Source: CAD feature listing. Evaluate the final solid. Frame: model axes, mm. A direction names the side the tool comes from. Give positions to 0.01 mm unless a question says otherwise; leave off trailing zeros. Order: outer loops, then holes, each group sorted by start corner. A loop starts at its lowest first (then second) coordinate and runs counter-clockwise, first axis right, second up.
from build123d import *

# Parameters (mm, degrees)
SKETCH1_W           = 50
SKETCH1_H           = 90
BOSS_EXTRUDE1_DEPTH = 10
SKETCH2_W           = 50
SKETCH2_H           = 50
SKETCH2_R           = 4.25
BOSS_EXTRUDE2_DEPTH = 10
SKETCH3_R           = 8.5
CUT_EXTRUDE1_DEPTH  = 5
CHAMFER1_SIZE       = 2


with BuildPart() as part:
    # Sketch1 → Boss-Extrude1 (new body)
    with BuildSketch(Plane(origin=(0, 0, 0), x_dir=(1, 0, 0), z_dir=(0, 1, 0))):
        with Locations((25, 45)):
            Rectangle(SKETCH1_W, SKETCH1_H)
        with BuildLine():
            Line((9, 6), (9, 84))
            ThreePointArc((9, 84), (12, 87), (15, 84))
            Line((15, 84), (15, 6))
            ThreePointArc((15, 6), (12, 3), (9, 6))
        make_face(mode=Mode.SUBTRACT)
        with BuildLine():
            Line((35, 6), (35, 84))
            ThreePointArc((35, 84), (38, 87), (41, 84))
            Line((41, 84), (41, 6))
            ThreePointArc((41, 6), (38, 3), (35, 6))
        make_face(mode=Mode.SUBTRACT)
    extrude(amount=BOSS_EXTRUDE1_DEPTH)

    # Sketch2 → Boss-Extrude2 (add)
    with BuildSketch(Plane.XY):
        with Locations((25, 25)):
            Rectangle(SKETCH2_W, SKETCH2_H)
        with Locations((25, 40)):
            Circle(SKETCH2_R, mode=Mode.SUBTRACT)
        with Locations((25, 20)):
            Circle(SKETCH2_R, mode=Mode.SUBTRACT)
    extrude(amount=BOSS_EXTRUDE2_DEPTH)

    # Sketch3 → Cut-Extrude1 (cut)
    with BuildSketch(Plane(origin=(0, 0, 0), x_dir=(-1, 0, 0), z_dir=(0, 0, -1))):
        with Locations((-25, 40)):
            Circle(SKETCH3_R)
        with Locations((-25, 20)):
            Circle(SKETCH3_R)
    extrude(amount=-CUT_EXTRUDE1_DEPTH, mode=Mode.SUBTRACT)

    # Chamfer1
    # the kernel refuses this chamfer: 2 mm, written as the material it takes off along each edge
    with BuildSketch(Plane(origin=(50, 10, 0), x_dir=(0.027495876610585623, -0.9996219169112968, 0), z_dir=(0, 0, -1))) as chamfer1_piece_1:
        Polygon((CHAMFER1_SIZE * 0.999621916911, CHAMFER1_SIZE * 0.0274958766106), (-CHAMFER1_SIZE * 0.0274958766106, CHAMFER1_SIZE * 0.999621916911), (0, 0), align=None)
    extrude(amount=95.143365976, mode=Mode.SUBTRACT)
    with BuildSketch(Plane(origin=(55.143365976, 10, -90), x_dir=(0, -0.9996219169112968, -0.027495876610589075), z_dir=(-1, 0, 0)), Plane(origin=(-5.143365976, 50, 0), x_dir=(0, 0.02749587661058563, 0.9996219169112968), z_dir=(1, 0, 0))) as chamfer1_piece_2:
        Polygon((CHAMFER1_SIZE * 0.999621916911, CHAMFER1_SIZE * 0.0274958766106), (-CHAMFER1_SIZE * 0.0274958766106, CHAMFER1_SIZE * 0.999621916911), (0, 0), align=None)
    extrude(amount=60.286731952, mode=Mode.SUBTRACT)
    with BuildSketch(Plane(origin=(50, 55.143365976, 0), x_dir=(0.02749587661058563, 0, 0.9996219169112968), z_dir=(0, -1, 0))) as chamfer1_piece_3:
        Polygon((CHAMFER1_SIZE * 0.999621916911, CHAMFER1_SIZE * 0.0274958766106), (-CHAMFER1_SIZE * 0.0274958766106, CHAMFER1_SIZE * 0.999621916911), (0, 0), align=None)
    extrude(amount=45.143365976, mode=Mode.SUBTRACT)
    with BuildSketch(Plane(origin=(0, 10, 0), x_dir=(0.9996219169112968, 0, -0.027495876610586372), z_dir=(0, 1, 0))) as chamfer1_piece_4:
        Polygon((CHAMFER1_SIZE * 0.999621916911, -CHAMFER1_SIZE * 0.0274958766106), (-CHAMFER1_SIZE * 0.0274958766106, -CHAMFER1_SIZE * 0.999621916911), (0, 0), align=None)
    extrude(amount=45.143365976, mode=Mode.SUBTRACT)
    with BuildSketch(Plane(origin=(0, 10, -95.143365976), x_dir=(0.9996219169112968, 0.027495876610586494, 0), z_dir=(0, 0, 1))) as chamfer1_piece_5:
        Polygon((CHAMFER1_SIZE * 0.999621916911, -CHAMFER1_SIZE * 0.0274958766106), (-CHAMFER1_SIZE * 0.0274958766106, -CHAMFER1_SIZE * 0.999621916911), (0, 0), align=None)
    extrude(amount=95.143365976, mode=Mode.SUBTRACT)
    with BuildSketch(Plane(origin=(50, 55.143365976, 0), x_dir=(0.02749587661058563, 0, 0.9996219169112968), z_dir=(0, -1, 0))) as chamfer1_piece_6a_section:
        Polygon((CHAMFER1_SIZE * 0.999621916911, CHAMFER1_SIZE * 0.0274958766106), (-CHAMFER1_SIZE * 0.0274958766106, CHAMFER1_SIZE * 0.999621916911), (0, 0), align=None)
    chamfer1_piece_6a = extrude(amount=50.286731952, mode=Mode.PRIVATE)
    chamfer1_piece_6a = split(chamfer1_piece_6a, bisect_by=Plane(origin=(49.340412746, 10, 0.659587254), z_dir=(0, -1, 0)), keep=Keep.TOP, mode=Mode.PRIVATE)
    with BuildSketch(Plane(origin=(50, 10, 5.143365976), x_dir=(0.027495876610585623, -0.9996219169112968, 0), z_dir=(0, 0, -1))) as chamfer1_piece_6b_section:
        Polygon((CHAMFER1_SIZE * 0.999621916911, CHAMFER1_SIZE * 0.0274958766106), (-CHAMFER1_SIZE * 0.0274958766106, CHAMFER1_SIZE * 0.999621916911), (0, 0), align=None)
    chamfer1_piece_6b = extrude(amount=100.286731952, mode=Mode.PRIVATE)
    chamfer1_piece_6b = split(chamfer1_piece_6b, bisect_by=Plane(origin=(49.340412746, 9.340412746, 0), z_dir=(0, 0, 1)), keep=Keep.TOP, mode=Mode.PRIVATE)
    chamfer1_piece_6 = chamfer1_piece_6a & chamfer1_piece_6b
    add(chamfer1_piece_6, mode=Mode.SUBTRACT)
    with BuildSketch(Plane(origin=(0, 4.856634024, 0), x_dir=(0.9996219169112968, 0, -0.027495876610586372), z_dir=(0, 1, 0))) as chamfer1_piece_7a_section:
        Polygon((CHAMFER1_SIZE * 0.999621916911, -CHAMFER1_SIZE * 0.0274958766106), (-CHAMFER1_SIZE * 0.0274958766106, -CHAMFER1_SIZE * 0.999621916911), (0, 0), align=None)
    chamfer1_piece_7a = extrude(amount=50.286731952, mode=Mode.PRIVATE)
    chamfer1_piece_7a = split(chamfer1_piece_7a, bisect_by=Plane(origin=(0.659587254, 10, 0.659587254), z_dir=(0, -1, 0)), keep=Keep.TOP, mode=Mode.PRIVATE)
    with BuildSketch(Plane(origin=(0, 10, -95.143365976), x_dir=(0.9996219169112968, 0.027495876610586494, 0), z_dir=(0, 0, 1))) as chamfer1_piece_7b_section:
        Polygon((CHAMFER1_SIZE * 0.999621916911, -CHAMFER1_SIZE * 0.0274958766106), (-CHAMFER1_SIZE * 0.0274958766106, -CHAMFER1_SIZE * 0.999621916911), (0, 0), align=None)
    chamfer1_piece_7b = extrude(amount=100.286731952, mode=Mode.PRIVATE)
    chamfer1_piece_7b = split(chamfer1_piece_7b, bisect_by=Plane(origin=(0.659587254, 9.340412746, 0), z_dir=(0, 0, 1)), keep=Keep.TOP, mode=Mode.PRIVATE)
    chamfer1_piece_7 = chamfer1_piece_7a & chamfer1_piece_7b
    add(chamfer1_piece_7, mode=Mode.SUBTRACT)


solid = part.part
1) First-contact query: pin 1 Ø10 at (x, y) = (25, 40) entering from +Z; pin 2 Ø14 at (x, z) = (27, -49.5) entering from +Y; pin 3 Ø8.5 at (x, y) = (22.5, 22.5) entering from -Z; pin 4 Ø5 at (y, z) = (11, -16.5) entering from -X. Flat tips, straight axial feed; report the tip coordinate or a pass-through.
Checks:
pin 1: stops at z = 10
pin 2: stops at y = 10
pin 3: stops at z = 5
pin 4: stops at x = 0.5
2) Reachability of faces 5 (the face through (38, 5, -3)), 6 (the face through (26.84, 11.7, 2.46)), 7 (the face through (25, 10, -45)) from +Z, -Z, +X, -X, +Y, -Y: full face, straight path, thin tool, end or side. Return the list, or none.
Checks:
face 5: +Y, -Y
face 6: -Z
face 7: -Z, +X, -X, +Y
3) Section query A-A on y = 5.5. Output: boundary loops of the cut face in (x, z), and give its area (3 significant figures).
Checks:
outline: (0, -90) - (50, -90) - (50, 10) - (0, 10) - close; hole (9, -84) arc R3 ccw to (15, -84) - (15, -6) arc R3 ccw to (9, -6) - close; hole (35, -84) arc R3 ccw to (41, -84) - (41, -6) arc R3 ccw to (35, -6) - close
area: 4,010 mm2
4) Ray query, L1, parallel to Y at x = 25, z = 6.4; L2, parallel to Y at x = 25, z = 2; L3, parallel to X at y = 40, z = 7. Return the intervals inside material, ascending.
Checks:
L1: y = 0 to 15.75, 24.25 to 35.75, 44.25 to 50
L2: y = 0 to 11.5, 28.5 to 31.5, 48.5 to 50
L3: x = 0 to 20.75, 29.25 to 50
5) Section query C-C on z = -71. Output: boundary loops of the cut face in (x, y), and give its area (3 significant figures).
Checks:
outline: (0, 0) - (9, 0) - (9, 10) - (2, 10) - (0, 8) - close; (15, 0) - (35, 0) - (35, 10) - (15, 10) - close; (41, 0) - (50, 0) - (50, 8) - (48, 10) - (41, 10) - close
area: 376 mm2
6) Section query B-B on x = 38. Output: boundary loops of the cut face in (y, z), and give its area (3 significant figures).
Checks:
outline: (0, -90) - (8, -90) - (10, -88) - (10, -87) - (0, -87) - close; (0, -3) - (10, -3) - (10, 0) - (48, 0) - (50, 2) - (50, 10) - (0, 10) - close
area: 556 mm2
7) Section query D-D on x = 25. Output: boundary loops of the cut face in (y, z), and give its area (3 significant figures).
Checks:
outline: (0, -90) - (8, -90) - (10, -88) - (10, 0) - (11.5, 0) - (11.5, 5) - (15.75, 5) - (15.75, 10) - (0, 10) - close; (24.25, 5) - (28.5, 5) - (28.5, 0) - (31.5, 0) - (31.5, 5) - (35.75, 5) - (35.75, 10) - (24.25, 10) - close; (44.25, 5) - (48.5, 5) - (48.5, 0.5) - (50, 2) - (50, 10) - (44.25, 10) - close
area: 1,140 mm2
8) Pull-direction query (X, two-part tool) for faces 1 (the face through (49, 29, 1)), 2 (the face through (25, 49, 1)), 3 (the face through (1, 29, 1)), 4 (the face through (38, 5, -87)); classes: +X half, -X half, draft (parallel to the pull), parting line (faces both ways), or undercut.
Checks:
face 1: +X half
face 2: draft
face 3: -X half
face 4: undercut
